Here's how the part is built. I have some questions about the finished solid (model axes, mm). Face numbers are marked on the shaded views. Coordinates: 2 decimals unless noted, no trailing zeros. Write each loop counter-clockwise with the first axis right and the second up, starting at its lowest first coordinate (ties: lowest second). Pieces come first, ordered by that corner, then holes. Notation, with made-up numbers: (48, 12.5) -> (81, 12.5) arc R25 ccw to (81, 38.5) -> close; hole circle Ø3 at (34, 21.25). An arc over 180 degrees is marked (long way). Put each result on its own line as item: value.
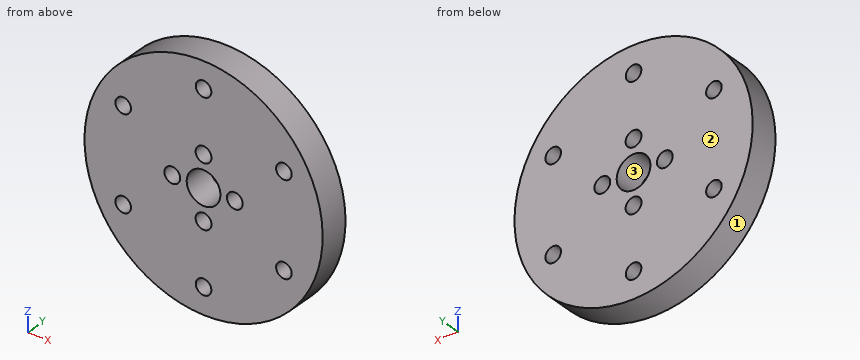
```python
from build123d import *

# Parameters (mm, degrees)
SKETCH1_R           = 30.48
BOSS_EXTRUDE1_DEPTH = 7.62
SKETCH2_R           = 1.9939
CUT_EXTRUDE1_DEPTH  = 44.773567367
CIRPATTERN1_COUNT   = 6
SKETCH3_R           = 4.318
SKETCH3_R_2         = 2.032
CUT_EXTRUDE2_DEPTH  = 44.773567367
CIRPATTERN2_COUNT   = 4


with BuildPart() as part:
    # Sketch1 → Boss-Extrude1 (new body)
    with BuildSketch(Plane(origin=(0, 0, 0), x_dir=(1, 0, 0), z_dir=(0, 1, 0))):
        with Locations(Location((0, 0, 0), (0, 0, 90))):
            Circle(SKETCH1_R)
    extrude(amount=BOSS_EXTRUDE1_DEPTH)

    # Sketch2 → Cut-Extrude1 (cut, through all)
    with BuildSketch(Plane(origin=(0, 7.62, 0), x_dir=(1, 0, 0), z_dir=(0, 1, 0))):
        with Locations(Location((0, -23.749, 0), (0, 0, 270))):
            Circle(SKETCH2_R)
    cut_extrude1 = extrude(amount=-CUT_EXTRUDE1_DEPTH, mode=Mode.SUBTRACT)

    # CirPattern1: Cut-Extrude1 ×6 about axis
    cirpattern1_axis = Axis((0, 0, 0), (0, 1, 0))
    for i in range(1, CIRPATTERN1_COUNT):
        add(cut_extrude1.rotate(cirpattern1_axis, i * 360 / CIRPATTERN1_COUNT), mode=Mode.SUBTRACT)

    # Sketch3 → Cut-Extrude2 (cut, through all)
    with BuildSketch(Plane(origin=(0, 7.62, 0), x_dir=(1, 0, 0), z_dir=(0, 1, 0))):
        with Locations(Location((0, 0, 0), (0, 0, 270))):
            Circle(SKETCH3_R)
        with Locations(Location((0, -8.001, 0), (0, 0, 270))):
            Circle(SKETCH3_R_2)
    cut_extrude2 = extrude(amount=-CUT_EXTRUDE2_DEPTH, mode=Mode.SUBTRACT)

    # CirPattern2: Cut-Extrude2 ×4 about axis
    cirpattern2_axis = Axis((0, 0, 0), (0, 1, 0))
    for i in range(1, CIRPATTERN2_COUNT):
        add(cut_extrude2.rotate(cirpattern2_axis, i * 360 / CIRPATTERN2_COUNT), mode=Mode.SUBTRACT)


solid = part.part
```
Item 1: Imagine slicing it at C-C on z = -8. Write out the boundary of the cut face in (x, y), then the cut area to 3 significant figures.
Output:
outline: (-29.41, 0) -> (-2.03, 0) -> (-2.03, 7.62) -> (-29.41, 7.62) -> close; (2.03, 0) -> (29.41, 0) -> (29.41, 7.62) -> (2.03, 7.62) -> close
area: 417 mm²
Item 2: If we mould it in two halves opening along X, with no side actions, what happens to the marked faces 1, 2 and 3? For each: released by +X, released by -X, zero draft, split by the parting line, or undercut.
Output:
face 1: split by the parting line
face 2: zero draft
face 3: undercut
Item 3: Imagine slicing it at A-A on z = 0. Write out the boundary of the cut face in (x, y).
Output:
outline: (-30.48, 0) -> (-10.03, 0) -> (-10.03, 7.62) -> (-30.48, 7.62) -> close; (-5.97, 0) -> (-4.32, 0) -> (-4.32, 7.62) -> (-5.97, 7.62) -> close; (4.32, 0) -> (5.97, 0) -> (5.97, 7.62) -> (4.32, 7.62) -> close; (10.03, 0) -> (30.48, 0) -> (30.48, 7.62) -> (10.03, 7.62) -> close
Item 4: Imagine slicing it at D-D on x = 0. Write out the boundary of the cut face in (y, z), then the cut area to 3 significant figures.
Output:
outline: (0, -30.48) -> (7.62, -30.48) -> (7.62, -25.74) -> (0, -25.74) -> close; (0, -21.76) -> (7.62, -21.76) -> (7.62, -10.03) -> (0, -10.03) -> close; (0, -5.97) -> (7.62, -5.97) -> (7.62, -4.32) -> (0, -4.32) -> close; (0, 4.32) -> (7.62, 4.32) -> (7.62, 5.97) -> (0, 5.97) -> close; (0, 10.03) -> (7.62, 10.03) -> (7.62, 21.76) -> (0, 21.76) -> close; (0, 25.74) -> (7.62, 25.74) -> (7.62, 30.48) -> (0, 30.48) -> close
area: 276 mm²
Item 5: For P1, Ø1, axis at x = 8, y = 7, coming from the -Z side; P2, Ø4, axis at y = 4, z = -5, coming from the -X side; P3, Ø1.5, axis at y = 2.5, z = 16, coming from the +X side, each with a flat end and sliding along its axis, tell me the tip position at first contact or that it passes through.
Output:
P1: stops at z = -29.54
P2: stops at x = -30.33
P3: stops at x = 26.39
Item 6: Please list where these lines run through material, in increasing order: line 1 along Z through (x, y) = (-22, 3.25); line 2 along X through (y, z) = (5, 24); line 3 along X through (y, z) = (6, -3). Write a range as from..to.
Output:
line 1: z = -21.1..-13.26, -10.49..10.49, 13.26..21.1
line 2: x = -18.79..-1.98, 1.98..18.79
line 3: x = -30.33..-3.11, 3.11..30.33
Item 7: Imagine slicing it at B-B on x = 19.5. Write out the boundary of the cut face in (y, z).
Output:
outline: (0, -23.43) -> (7.62, -23.43) -> (7.62, -13.56) -> (0, -13.56) -> close; (0, -10.19) -> (7.62, -10.19) -> (7.62, 10.19) -> (0, 10.19) -> close; (0, 13.56) -> (7.62, 13.56) -> (7.62, 23.43) -> (0, 23.43) -> close
